Can you work these out from the model? Positions are in its coordinate system, mm. A direction names the side the tool comes from. Coordinates: 2 decimals unless noted, no trailing zeros. Order: outer loops, then holes, each group sorted by start corner. A loop starts at its lowest first (then second) coordinate and runs counter-clockwise, first axis right, second up. Notation, with made-up numbers: (56.25, -0.75) -> (115.25, -0.75) arc R13 ccw to (115.25, 16.25) -> close; hole circle Ø11 at (6.25, -1.5). An arc over 180 degrees is marked (long way). Answer as a JSON object with one key per item and string values. Group by question number.
(1) If we mould it in two halves opening along X, with no side actions, what happens to faces 1 (the flat face through (25, -37, 3)), 2 (the flat face through (-6.084, -10.344, 3.768)), 3 (the flat face through (12, 1, 0))? For each: pulls with the +X half, pulls with the -X half, needs draft (parallel to the pull), parting line crosses it, or undercut.
(2) I want a section at D-D, the plane z = 3.85. State how many separate pieces and enclosed holes the cut face has, plus the area to 3 significant figures.
(3) I want a section at B-B, the plane x = 17. List the corners of the cut face in (y, z) for me, plus the area to 3 significant figures.
(4) Which directions (+Z, -Z, +X, -X, +Y, -Y) give clear straight access to the entire face, cutting with the end or side of a thin tool? Please do faces 4 (the flat face through (-25, 36, 3)), 5 (the cylindrical face through (11.84, 60.74, 2.83)), 6 (the flat face through (-6, -6, 2.5)).
(5) I want a section at C-C, the plane y = 0. List the corners of the cut face in (x, z) for me, plus the area to 3 significant figures.
(6) For pin 1 (3 mm diameter, centred on x = 0, y = -10, fed in from -Z); pin 2 (7 mm diameter, centred on x = -4.5, y = 3.5, fed in from +Z); pin 3 (3.5 mm diameter, centred on x = 17, y = 46, fed in from -Z), each with a flat end and sliding along its axis, tell me the tip position at first contact or that it passes through.
(7) I want a section at A-A, the plane y = 59.5. List the corners of the cut face in (x, z) for me, plus the area to 3 significant figures.
(8) I need wall thicknesses on line 1 (Y direction, x = -17, z = 3.7); line 2 (X direction, y = -59.5, z = 2.05); line 3 (Y direction, x = -10, z = 4.35). Which ranges of each line are inside material? Lowest first, please.
from build123d import *

# Parameters (mm, degrees)
SKETCH_1_W          = 50
SKETCH_1_H          = 140
EXTRUDE_1_DEPTH     = 5
SKETCH_16_R         = 3
EXTRUDE_2_DEPTH     = 5
CUT_EXTRUDE_5_DEPTH = 2.5
SKETCH_12_R         = 7.5
CUT_EXTRUDE_6_DEPTH = 2.5
SKETCH_13_R         = 1.25
CUT_EXTRUDE_7_DEPTH = 76.557924799
FILLET_2_R          = 10
FILLET_1_R          = 5
SKETCH_14_R         = 1
SKETCH_14_R_2       = 1.6
SKETCH_14_R_3       = 1.25
CUT_EXTRUDE_8_DEPTH = 76.557924799
CHAMFER_1_SIZE      = 0.6


with BuildPart() as part:
    # 草图1 → 凸台-拉伸1 (new body)
    with BuildSketch(Plane.XY):
        Rectangle(SKETCH_1_W, SKETCH_1_H)
    extrude(amount=EXTRUDE_1_DEPTH)

    # 草图16 → 凸台-拉伸2 (add)
    with BuildSketch(Plane.XY.offset(5)):
        with Locations((25, 0)):
            Circle(SKETCH_16_R)
        with Locations((-25, 0)):
            Circle(SKETCH_16_R)
    extrude(amount=-EXTRUDE_2_DEPTH)

    # 草图11 → 切除-拉伸5 (cut)
    with BuildSketch(Plane.XY.offset(5)):
        Polygon((0, 13.856406461), (-12, 6.92820323), (-12, -6.92820323), (0, -13.856406461), (12, -6.92820323), (12, 6.92820323), align=None)
    extrude(amount=-CUT_EXTRUDE_5_DEPTH, mode=Mode.SUBTRACT)

    # 草图12 → 切除-拉伸6 (cut)
    with BuildSketch(Plane.XY.offset(2.5)):
        Circle(SKETCH_12_R)
    extrude(amount=-CUT_EXTRUDE_6_DEPTH, mode=Mode.SUBTRACT)

    # 草图13 → 切除-拉伸7 (cut, through all)
    with BuildSketch(Plane.XY.offset(5)):
        with Locations((25, 0)):
            Circle(SKETCH_13_R)
        with Locations(Location((-25, 0, 0), (0, 0, 180))):
            Circle(SKETCH_13_R)
    extrude(amount=-CUT_EXTRUDE_7_DEPTH, mode=Mode.SUBTRACT)

    # 圆角2
    fillet_2_edges = [part.edges().sort_by_distance(p)[0] for p in [
        (25, -3, 2.5),
        (25, 3, 2.5),
        (-25, 3, 2.5),
        (-25, -3, 2.5),
    ]]
    fillet(fillet_2_edges, radius=FILLET_2_R)

    # 圆角1
    fillet_1_edges = [part.edges().sort_by_distance(p)[0] for p in [
        (25, -70, 2.5),
        (-25, -70, 2.5),
        (-25, 70, 2.5),
        (25, 70, 2.5),
    ]]
    fillet(fillet_1_edges, radius=FILLET_1_R)

    # 草图14 → 切除-拉伸8 (cut, through all)
    with BuildSketch(Plane.XY.offset(5)):
        with Locations((0, 10)):
            Circle(SKETCH_14_R)
        with Locations((0, 25)):
            Circle(SKETCH_14_R)
        with Locations((0, 40)):
            Circle(SKETCH_14_R)
        with Locations((17, 46)):
            Circle(SKETCH_14_R_2)
        with Locations(Location((-17, 46, 0), (0, 0, 180))):
            Circle(SKETCH_14_R_2)
        with Locations((-5, 59.5)):
            Circle(SKETCH_14_R_3)
        with Locations((12, 59.5)):
            Circle(SKETCH_14_R_3)
    cut_extrude_8 = extrude(amount=-CUT_EXTRUDE_8_DEPTH, mode=Mode.SUBTRACT)

    # 镜向1: 切除-拉伸8 across plane
    add(cut_extrude_8.mirror(Plane.ZX), mode=Mode.SUBTRACT)

    # 倒角1
    chamfer_1_edges = [part.edges().sort_by_distance(p)[0] for p in [
        (25, -36.653311931, 0),
        (0, -70, 0),
        (23.535533906, 68.535533906, 0),
        (23.535533906, -68.535533906, 0),
        (-23.535533906, -68.535533906, 0),
        (-23.535533906, 68.535533906, 0),
        (-1, 10, 0),
        (-15.4, 46, 0),
        (-1, 40, 0),
        (-1, 25, 0),
        (15.4, 46, 0),
        (-6.25, 59.5, 0),
        (10.75, 59.5, 0),
        (-1, -10, 0),
        (-15.4, -46, 0),
        (-1, -40, 0),
        (-1, -25, 0),
        (15.4, -46, 0),
        (-6.25, -59.5, 0),
        (10.75, -59.5, 0),
        (-7.5, 0, 0),
        (23.75, 0, 0),
        (-23.75, 0, 0),
        (-25, -36.653311931, 0),
        (-28, 0, 0),
        (28, 0, 0),
        (25, 36.653311931, 0),
        (-25.594600569, -4.90979276, 0),
        (-25.594600569, 4.90979276, 0),
        (25.594600569, -4.90979276, 0),
        (25.594600569, 4.90979276, 0),
        (-25, 36.653311931, 0),
        (0, 70, 0),
    ]]
    chamfer(chamfer_1_edges, length=CHAMFER_1_SIZE)


solid = part.part
Computed values:
{
 "1": {"face 1": "pulls with the +X half", "face 2": "undercut", "face 3": "needs draft"},
 "2": {"separate pieces": "1", "enclosed holes": "15", "area": "6,450 mm2"},
 "3": {"outline": "(-70, 0.6) -> (-69.4, 0) -> (-48.2, 0) -> (-47.6, 0.6) -> (-47.6, 5) -> (-70, 5) -> close; (-44.4, 0.6) -> (-43.8, 0) -> (43.8, 0) -> (44.4, 0.6) -> (44.4, 5) -> (-44.4, 5) -> close; (47.6, 0.6) -> (48.2, 0) -> (69.4, 0) -> (70, 0.6) -> (70, 5) -> (47.6, 5) -> close", "area": "667 mm2"},
 "4": {"face 4": "+Z, -Z, -X, +Y", "face 5": "+Z, -Z", "face 6": "+Z"},
 "5": {"outline": "(-28, 0.6) -> (-27.4, 0) -> (-26.85, 0) -> (-26.25, 0.6) -> (-26.25, 5) -> (-28, 5) -> close; (-23.75, 0.6) -> (-23.15, 0) -> (-8.1, 0) -> (-7.5, 0.6) -> (-7.5, 2.5) -> (-12, 2.5) -> (-12, 5) -> (-23.75, 5) -> close; (7.5, 0.6) -> (8.1, 0) -> (23.15, 0) -> (23.75, 0.6) -> (23.75, 5) -> (12, 5) -> (12, 2.5) -> (7.5, 2.5) -> close; (26.25, 0.6) -> (26.85, 0) -> (27.4, 0) -> (28, 0.6) -> (28, 5) -> (26.25, 5) -> close", "area": "156 mm2"},
 "6": {"pin 1": "stops at z = 0.1", "pin 2": "stops at z = 2.5", "pin 3": "stops at z = 0.45"},
 "7": {"outline": "(-25, 0.6) -> (-24.4, 0) -> (-6.85, 0) -> (-6.25, 0.6) -> (-6.25, 5) -> (-25, 5) -> close; (-3.75, 0.6) -> (-3.15, 0) -> (10.15, 0) -> (10.75, 0.6) -> (10.75, 5) -> (-3.75, 5) -> close; (13.25, 0.6) -> (13.85, 0) -> (24.4, 0) -> (25, 0.6) -> (25, 5) -> (13.25, 5) -> close", "area": "224 mm2"},
 "8": {"line 1": "y = -70 to -47.6, -44.4 to 44.4, 47.6 to 70", "line 2": "x = -25 to -6.25, -3.75 to 10.75, 13.25 to 25", "line 3": "y = -70 to -8.08, 8.08 to 70"}
}
